Here's how the part is built. I have some questions about the finished solid (model axes, mm). Give positions to 0.01 mm unless a question says otherwise; leave off trailing zeros. Write each loop counter-clockwise with the first axis right and the second up, starting at its lowest first coordinate (ties: lowest second). Pieces come first, ordered by that corner, then holes. Notation, with made-up numbers: (49, 31) - (57, 31) arc R27 ccw to (57, 69) - close; hole circle Ø3 at (81.25, 52.25). An arc over 180 degrees is marked (long way). Write each question's results on one line, items separated by ' | '. Start each with the question number.
Item 1: Suppose I cut it at A-A on z = 0.85. Count the separate pieces of the cut face and the enclosed holes in it, then the cut area to 3 significant figures.
Item 2: Suppose I cut it at C-C on x = 349. List the corners of the cut face in (y, z) for me.
Item 3: Please list where these lines run through material, in increasing order: line 1 along X through (y, z) = (5, 0.65); line 2 along X through (y, z) = (108, 0.15); line 3 along Y through (x, z) = (372, 1).
Item 4: Suppose I cut it at B-B on y = 135. List the corners of the cut face in (x, z) for me.
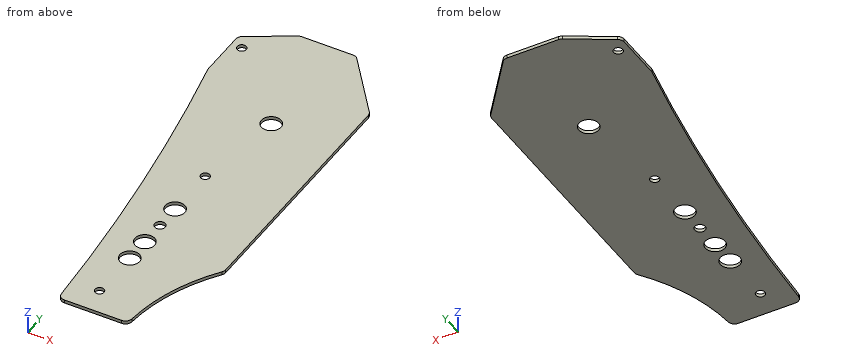
Autodesk Inventor part; units mm, degrees
ref_plane "YZ Plane" through (0, 0, 0) normal (1, 0, 0) x (0, 1, 0)
ref_plane "XZ Plane" through (0, 0, 0) normal (0, 1, 0) x (-1, 0, 0)
ref_plane "XY Plane" through (0, 0, 0) normal (0, 0, 1) x (1, 0, 0)
sketch "Sketch1" plane through (0, 0, 0) normal (0, 0, 1) x (1, 0, 0)
  line L0 (377.0029, 160.9063) -> (356.3654, 160.9063)
  circle A0 centre (336.9408, 141.8563) radius 2.1844
  line L1 (331.7592, 123.8223) -> (331.7592, 147.1903)
  line L2 (331.7592, 147.1903) -> (332.7752, 148.2063)
  line L3 (332.7752, 148.2063) -> (342.0779, 148.2063)
  line L4 (356.3654, 160.9063) -> (353.9842, 160.9063)
  line L5 (354.8564, 160.9063) -> (379.7418, 160.9063)
  line L6 (382.24, 159.6907) -> (404.7811, 130.9525)
  line L7 (405.4579, 128.993) -> (405.4579, 8.9191)
  line L8 (353.2344, 160.4607) -> (333.3122, 148.6212)
  line L9 (331.7592, 145.8918) -> (331.7592, 122.4835)
  arc A1 (404.8445, 7.0432) -> (387.8405, -39.3429) centre (476.7839, -45.6377) ccw
  line L10 (384.6734, -42.2937) -> (356.983, -42.2937)
  arc A2 (353.8134, -39.3043) -> (331.7592, 122.4835) centre (-705.6943, -101.3347) ccw
  arc A3 (333.3122, 148.6212) -> (331.7592, 145.8918) centre (334.9342, 145.8918) ccw
  arc A4 (354.8564, 160.9063) -> (353.2344, 160.4607) centre (354.8564, 157.7313) ccw
  arc A5 (382.24, 159.6907) -> (379.7418, 160.9063) centre (379.7418, 157.7313) ccw
  arc A6 (405.4579, 128.993) -> (404.7811, 130.9525) centre (402.2829, 128.993) ccw
  arc A7 (404.8445, 7.0432) -> (405.4579, 8.9191) centre (402.2829, 8.9191) ccw
  arc A8 (384.6734, -42.2937) -> (387.8405, -39.3429) centre (384.6734, -39.1187) ccw
  arc A9 (353.8134, -39.3043) -> (356.983, -42.2937) centre (356.983, -39.1187) ccw
  circle A10 centre (373.0342, 103.7563) radius 4.7625
  circle A11 centre (366.6842, 59.3063) radius 2.1844
  circle A12 centre (366.6842, 21.2063) radius 2.54
  circle A13 centre (366.6842, 33.9063) radius 4.7625
  circle A14 centre (366.6842, 8.5063) radius 4.7625
  circle A15 centre (366.6842, -4.1937) radius 4.7625
  circle A16 centre (366.6842, -29.5937) radius 2.1844
  point P0 (0, 0)
  point P1 (405.4579, 7.8708)
  point P2 (387.6807, -42.2937)
  point P3 (353.9842, -42.2937)
  dimension "d1" = 3.175
  dimension "d2" = 3.175
  dimension "d3" = 9.525
  dimension "d4" = 4.3688
  dimension "d5" = 5.08
  dimension "d6" = 9.525
  dimension "d7" = 9.525
  dimension "d8" = 9.525
  dimension "d9" = 4.3688
extrude "Extrusion1" add sketch "Sketch1" along normal blind 1.5875 contours L5 A5 L6 A6 L7 A7 A1 A8 L10 A9 A2 L9 L1 A3 L8 A4 L4 L0
Checked values:
1) separate pieces: 1 | enclosed holes: 8 | area: 11,300 mm^2
2) outline: (17.09, 0) - (157.94, 0) - (157.94, 1.59) - (17.09, 1.59) - close
3) line 1: x = 350.29 to 363.46, 369.91 to 403.39 | line 2: x = 334.78 to 370.87, 375.2 to 405.46 | line 3: y = -42.29 to 99.11, 108.41 to 160.91
4) outline: (331.76, 0) - (401.61, 0) - (401.61, 1.59) - (331.76, 1.59) - close
